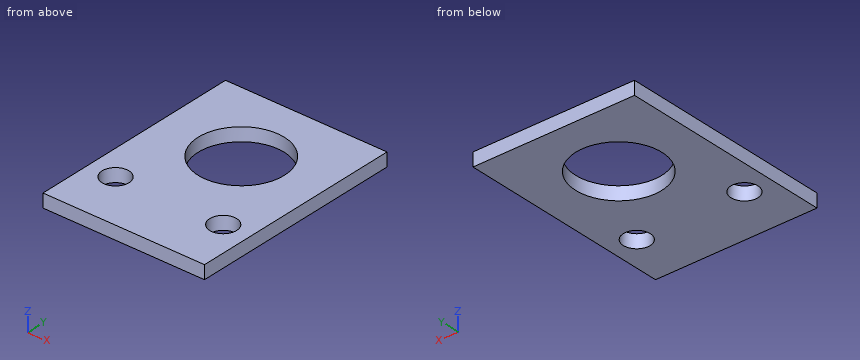
```python
from build123d import *

# Parameters (mm, degrees)
SKETCH1_W           = 60
SKETCH1_H           = 80
SKETCH1_R           = 16
SKETCH1_R_2         = 5
BOSS_EXTRUDE1_DEPTH = 5


with BuildPart() as part:
    # Sketch1 → Boss-Extrude1 (new body)
    with BuildSketch(Plane.XY):
        Rectangle(SKETCH1_W, SKETCH1_H)
        with Locations((0, 11.5)):
            Circle(SKETCH1_R, mode=Mode.SUBTRACT)
        with Locations((20, -20)):
            Circle(SKETCH1_R_2, mode=Mode.SUBTRACT)
        with Locations(Location((-20, -20, 0), (0, 0, 180))):
            Circle(SKETCH1_R_2, mode=Mode.SUBTRACT)
    extrude(amount=BOSS_EXTRUDE1_DEPTH)


solid = part.part
```
Can you work these out from the model? Positions are in its coordinate system, mm. Coordinates: 2 decimals unless noted, no trailing zeros. Write each loop counter-clockwise with the first axis right and the second up, starting at its lowest first coordinate (ties: lowest second). Pieces come first, ordered by that corner, then holes. Notation, with made-up numbers: (-7, 16.25) - (41, 16.25) arc R16 ccw to (41, 43.25) - close; hole circle Ø6 at (-10, -31.5). An arc over 180 degrees is marked (long way). Return JSON: item names as keys, results as strings.
Q1. I'm going to push a flat-ended pin straight in: pin 1 Ø16 at (x, y) = (20, -20) entering from -Z. Where does the tip first touch, or does it pass through?
Computed values:
{"pin 1": "stops at z = 0"}
Q2. If we section it at B-B (x = 0): Please give me the cut outline in (y, z).
Computed values:
{"outline": "(-40, 0) - (-4.5, 0) - (-4.5, 5) - (-40, 5) - close; (27.5, 0) - (40, 0) - (40, 5) - (27.5, 5) - close"}
Q3. If we section it at D-D (x = 20): Please give me the cut outline in (y, z), then the cut area to 3 significant figures.
Computed values:
{"outline": "(-40, 0) - (-25, 0) - (-25, 5) - (-40, 5) - close; (-15, 0) - (40, 0) - (40, 5) - (-15, 5) - close", "area": "350 mm2"}
Q4. If we section it at A-A (z = 3.2): Please give me the cut outline in (x, y).
Computed values:
{"outline": "(-30, -40) - (30, -40) - (30, 40) - (-30, 40) - close; hole circle Ø10 at (-20, -20); hole circle Ø32 at (0, 11.5); hole circle Ø10 at (20, -20)"}
Q5. Please list where these lines run through material, in increasing order: L1, parallel to X at y = 12, z = 4.3; L2, parallel to Y at x = 0, z = 2.9; L3, parallel to X at y = -24, z = 0.75. Write a range as from..to.
Computed values:
{"L1": "x = -30..-15.99, 15.99..30", "L2": "y = -40..-4.5, 27.5..40", "L3": "x = -30..-23, -17..17, 23..30"}
Q6. If we section it at C-C (y = -20): Please give me the cut outline in (x, z).
Computed values:
{"outline": "(-30, 0) - (-25, 0) - (-25, 5) - (-30, 5) - close; (-15, 0) - (15, 0) - (15, 5) - (-15, 5) - close; (25, 0) - (30, 0) - (30, 5) - (25, 5) - close"}
